Autodesk Inventor part; units mm, degrees
ref_plane "YZ Plane" through (0, 0, 0) normal (1, 0, 0) x (0, 1, 0)
ref_plane "XZ Plane" through (0, 0, 0) normal (0, 1, 0) x (-1, 0, 0)
ref_plane "XY Plane" through (0, 0, 0) normal (0, 0, 1) x (1, 0, 0)
sketch "Sketch1" plane through (0, 0, 0) normal (0, 1, 0) x (-1, 0, 0)
  line L0 (14.605, -25.4) -> (14.605, 25.4)
  line L1 (-14.605, -25.4) -> (-14.605, 25.4)
  line L2 (11.43, -28.575) -> (-11.43, -28.575)
  line L3 (11.43, 28.575) -> (-11.43, 28.575)
  arc A0 (11.43, -28.575) -> (14.605, -25.4) centre (11.43, -25.4) ccw
  arc A1 (-14.605, -25.4) -> (-11.43, -28.575) centre (-11.43, -25.4) ccw
  arc A2 (14.605, 25.4) -> (11.43, 28.575) centre (11.43, 25.4) ccw
  arc A3 (-11.43, 28.575) -> (-14.605, 25.4) centre (-11.43, 25.4) ccw
  point P0 (0, 0)
  dimension "d0" = 3.175
  dimension "d1" = 50.8
  dimension "d2" = 3.175
  dimension "d3" = 22.86
  dimension "d4" = 11.43
  dimension "d5" = 25.4
  dimension "d6" = 3.175
  dimension "d7" = 3.175
extrude "Extrusion1" add sketch "Sketch1" along normal blind 3.175
sketch "Sketch2" plane through (0, 3.175, 0) normal (0, 1, 0) x (1, 0, 0)
  line L0 (-13.208, 25.781) -> (-13.208, -25.781)
  line L1 (-14.605, 25.4) -> (-14.605, -25.4)
  arc A0 (-13.208, -25.781) -> (-11.811, -27.178) centre (-11.811, -25.781) ccw
  line L2 (-11.811, -27.178) -> (11.811, -27.178)
  line L3 (-11.43, -28.575) -> (11.43, -28.575)
  arc A1 (11.811, -27.178) -> (13.208, -25.781) centre (11.811, -25.781) ccw
  line L4 (13.208, -25.781) -> (13.208, 25.781)
  line L5 (14.605, -25.4) -> (14.605, 25.4)
  arc A2 (13.208, 25.781) -> (11.811, 27.178) centre (11.811, 25.781) ccw
  line L6 (11.811, 27.178) -> (-11.811, 27.178)
  arc A3 (-11.811, 27.178) -> (-13.208, 25.781) centre (-11.811, 25.781) ccw
  line L7 (-14.605, 25.4) -> (-14.605, -25.4)
  line L8 (-14.605, 25.4) -> (-14.605, -25.4)
  arc A4 (-14.605, -25.4) -> (-11.43, -28.575) centre (-11.43, -25.4) ccw
  arc A5 (-14.605, -25.4) -> (-11.43, -28.575) centre (-11.43, -25.4) ccw
  line L9 (-11.43, -28.575) -> (11.43, -28.575)
  arc A6 (11.43, -28.575) -> (14.605, -25.4) centre (11.43, -25.4) ccw
  arc A7 (11.43, -28.575) -> (14.605, -25.4) centre (11.43, -25.4) ccw
  line L10 (14.605, -25.4) -> (14.605, 25.4)
  arc A8 (14.605, 25.4) -> (11.43, 28.575) centre (11.43, 25.4) ccw
  line L11 (11.43, 28.575) -> (-11.43, 28.575)
  line L12 (-11.43, 28.575) -> (11.43, 28.575)
  arc A9 (-11.43, 28.575) -> (-14.605, 25.4) centre (-11.43, 25.4) ccw
  arc A10 (14.605, 25.4) -> (11.43, 28.575) centre (11.43, 25.4) ccw
  point P0 (0, 0)
  dimension "d10" = 1.397
  dimension "d11" = 1.397
  dimension "d12" = 1.397
  dimension "d14" = 1.397
  dimension "d15" = 1.397
  dimension "d16" = 1.397
  dimension "d17" = 1.397
  dimension "d18" = 1.397
extrude "Extrusion2" add sketch "Sketch2" along normal blind 17.78
sketch "Sketch4" plane through (-11.43, 0, 28.575) normal (0, 0, 1) x (1, 0, 0)
  line L0 (15.4305, 11.43) -> (7.4295, 11.43)
  line L1 (6.6675, 12.192) -> (6.6675, 20.955)
  line L2 (6.6675, 20.955) -> (16.1925, 20.955)
  line L3 (16.1925, 20.955) -> (16.1925, 12.192)
  line L4 (0, 20.955) -> (22.86, 20.955)
  line L5 (11.43, -2.422) -> (11.43, 18.2718) construction
  line L6 (22.86, 0) -> (22.86, 20.955) construction
  arc A0 (15.4019, 11.4305) -> (16.1925, 12.192) centre (15.4305, 12.192) ccw
  arc A1 (6.669, 12.2395) -> (7.4295, 11.43) centre (7.4295, 12.192) ccw
  point P0 (11.43, 0)
  dimension "d27" = 9.525
  dimension "d28" = 0
  dimension "d29" = 9.525
  dimension "d30" = 11.43
  dimension "d31" = 0.762
  dimension "d32" = 0.762
extrude "Extrusion3" cut sketch "Sketch4" against normal up to surface (1.397 mm away)
sketch "Sketch5" plane through (14.605, 0, 25.4) normal (1, 0, 0) x (0, 0, -1)
  line L0 (50.8, 20.955) -> (0, 20.955)
  line L1 (15.298, 9.091) -> (6.382, 9.091)
  line L2 (6.382, 9.091) -> (6.382, 20.955)
  line L3 (6.382, 20.955) -> (15.298, 20.955)
  line L4 (15.298, 20.955) -> (15.298, 9.091)
  line L5 (0, 0) -> (0, 20.955)
  line L6 (-3.175, 0) -> (-3.175, 20.955)
  point P0 (25.4, 0)
  point P1 (15.298, 20.955)
  dimension "d36" = 8.916
  dimension "d37" = 11.864
  dimension "d48" = 9.557
extrude "Extrusion4" cut sketch "Sketch5" against normal up to surface (1.397 mm away)
sketch "Sketch6" plane through (11.43, 0, -28.575) normal (0, 0, -1) x (-1, 0, 0)
  line L0 (23.241, 20.955) -> (-0.381, 20.955)
  line L1 (11.128, 20.955) -> (4.112, 20.955)
  line L2 (4.112, 20.955) -> (4.112, 11.582)
  line L3 (4.112, 11.582) -> (11.128, 11.582)
  line L4 (11.128, 11.582) -> (11.128, 20.955)
  line L5 (0, 0) -> (0, 20.955)
  circle A0 centre (11.43, 6.8195) radius 3.175
  line L6 (22.86, 0) -> (22.86, 20.955)
  line L7 (-3.175, 0) -> (-3.175, 20.955)
  point P0 (11.43, 0)
  dimension "d41" = 7.016
  dimension "d42" = 9.373
  dimension "d45" = 6.35
  dimension "d46" = 4.7625
  dimension "d47" = 11.43
  dimension "d49" = 7.287
extrude "Extrusion5" cut sketch "Sketch6" against normal up to surface (1.397 mm away)
fillet "Fillet1" radius 3.175 8 edges at (13.6751, 0, 27.6451) (14.605, 0, 0) (13.6751, 0, -27.6451) (0, 0, -28.575) (-13.6751, 0, -27.6451) (-14.605, 0, 0) (-13.6751, 0, 27.6451) (0, 0, 28.575)
properties part number "groundStation-top"
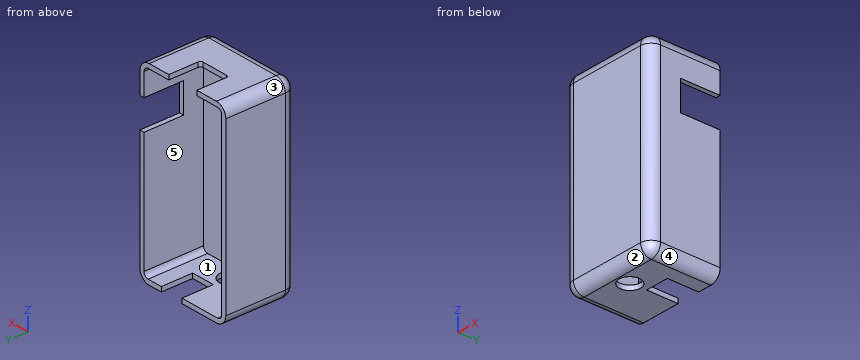
Can you work these out from the model? Positions are in its coordinate system, mm. Face numbers are marked on the shaded views. A direction names the side the tool comes from. Coordinates: 2 decimals unless noted, no trailing zeros. Loops run counter-clockwise (first coordinate to the right, second up) from the corner with the lowest first, then second, coordinate; pieces in that order, holes last. Notation, with made-up numbers: (58, 39.25) -> (108, 39.25) arc R13 cw to (108, 48.25) -> close; hole circle Ø6 at (61, -24.75). An arc over 180 degrees is marked (long way). Answer as a JSON object with one key per item and string values.
1) If I drill on line 1 (X direction, y = 17.75, z = -5.5) (3 decimals); line 2 (Z direction, x = 10.5, y = 13) (3 decimals); line 3 (Y direction, x = 10.5, z = 16.5) (3 decimals), over which ranges is the centre line in solid material (lowest first)?
Results:
{"line 1": "x = -14.605 to -13.208, 13.208 to 14.605", "line 2": "z = -28.575 to -27.178, 27.178 to 28.575", "line 3": "y = 0 to 3.175"}
2) Imagine slicing it at A-A (y = 17). Count the separate pieces of the cut face and the enclosed holes in it, then the cut area to 3 significant figures.
Results:
{"separate pieces": "3", "enclosed holes": "0", "area": "191 mm^2"}
3) Imagine slicing it at B-B (x = -1). Please give me the cut outline in (y, z) (3 decimals).
Results:
{"outline": "(0, -25.4) arc R3.175 ccw to (3.175, -28.575) -> (3.806, -28.575) -> (3.806, -27.178) -> (3.175, -27.178) -> (3.175, 27.178) -> (11.43, 27.178) -> (11.43, 28.575) -> (3.175, 28.575) arc R3.175 ccw to (0, 25.4) -> close; (9.833, -28.575) -> (20.955, -28.575) -> (20.955, -27.178) -> (9.833, -27.178) -> close"}
4) Imagine slicing it at D-D (x = -6.5). Please give me the cut outline in (y, z) (3 decimals), then the cut area to 3 significant figures.
Results:
{"outline": "(0, -25.4) arc R3.175 ccw to (3.175, -28.575) -> (20.955, -28.575) -> (20.955, -27.178) -> (3.175, -27.178) -> (3.175, 27.178) -> (20.955, 27.178) -> (20.955, 28.575) -> (3.175, 28.575) arc R3.175 ccw to (0, 25.4) -> close", "area": "227 mm^2"}
5) Imagine slicing it at C-C (z = -22). Please give me the cut outline in (x, y) (3 decimals), then the cut area to 3 significant figures.
Results:
{"outline": "(-14.605, 3.175) arc R3.175 ccw to (-11.43, 0) -> (11.43, 0) arc R3.175 ccw to (14.605, 3.175) -> (14.605, 20.955) -> (13.208, 20.955) -> (13.208, 3.175) -> (-13.208, 3.175) -> (-13.208, 20.955) -> (-14.605, 20.955) -> close", "area": "138 mm^2"}
6) Thinking about a two-plate mould opening in X: for the marked faces 1, 2 and 3, which applies, pulls with the +X half, pulls with the -X half, needs draft (parallel to the pull), parting line crosses it, or undercut?
Results:
{"face 1": "undercut", "face 2": "needs draft", "face 3": "pulls with the -X half"}
7) For the marked faces 4 and 5, which set-ups out of +Z, -Z, +X, -X, +Y, -Y let a thin tool reach every point of the face, with its end or its side?
Results:
{"face 4": "-Z, +X, +Y, -Y", "face 5": "+Y"}
8) For P1, Ø0.7, axis at x = 13.5, y = 14, coming from the -Z side; P2, Ø1.1, axis at x = 14, y = 17, coming from the +Z side; P3, Ø1.1, axis at x = 13.5, z = 14, coming from the +Y side, each with a flat end and sliding along its axis, tell me the tip position at first contact or that it passes through.
Results:
{"P1": "stops at z = -28.07", "P2": "stops at z = 27.85", "P3": "stops at y = 9.09"}
